Could you check a few things on this drawing? It's one solid part, dimensions in mm from its lowest x, y, z. A direction names the side the tool comes from. Round coordinates to 2 decimals unless told otherwise and drop trailing zeros. Write each loop counter-clockwise with the first axis right and the second up, starting at its lowest first coordinate (ties: lowest second). Pieces come first, ordered by that corner, then holes. Notation, with made-up numbers: (35.5, -7.5) -> (74.5, -7.5) arc R24 cw to (74.5, 6.5) -> close; hole circle Ø1 at (39.5, 48.25). An arc over 180 degrees is marked (long way). Answer in a Markdown table with one row per item. Add a question column.
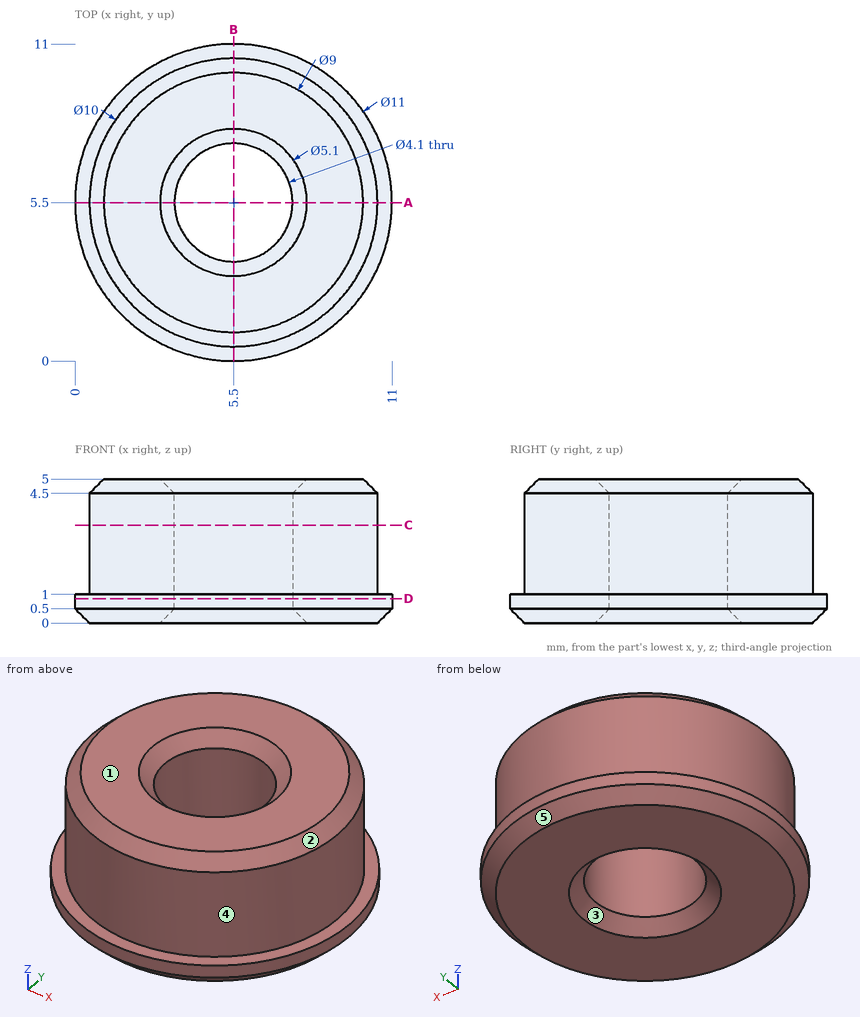
(1) I need wall thicknesses on L1, parallel to Y at x = 5.5, z = 1.6; L2, parallel to Y at x = 6.5, z = 4.4. Which ranges of each line are inside material? Lowest first, please.
(2) Suppose I cut it at A-A, the plane y = 5.5. Please give me the cut outline in (x, z), then the cut area to 3 significant figures.
(3) For P1, Ø1.5, axis at y = 7.5, z = 3.5, coming from the +X side; P2, Ø1.5, axis at y = 2.5, z = 3.5, coming from the +X side; P3, Ø2, axis at x = 4, z = 3, coming from the +Y side, each with a flat end and sliding along its axis, tell me the tip position at first contact or that it passes through.
(4) Suppose I cut it at C-C, the plane z = 3.4. Please give me the cut outline in (x, y).
(5) On a 3-axis mill with a long thin cutter (end or side, diameter ignored), from which of +Z, -Z, +X, -X, +Y, -Y can I reach the whole of each face in a straight line? I mean the marked faces 4 and 5. Say none if no direction works.
(6) If we mould it in two halves opening along Y, with no side actions, what happens to the marked faces 1, 2 and 3? For each: pulls with the +Y half, pulls with the -Y half, needs draft (parallel to the pull), parting line crosses it, or undercut.
(7) Suppose I cut it at D-D, the plane z = 0.85. Please give me the cut outline in (x, y), then the cut area to 3 significant figures.
Response:
| question | item | result |
|---|---|---|
| 1 | L1 | 0.5 to 3.45, 7.55 to 10.5 |
| 1 | L2 | 0.6 to 3.71, 7.29 to 10.4 |
| 2 | outline | (0, 0.5) -> (0.5, 0) -> (2.95, 0) -> (3.45, 0.5) -> (3.45, 4.5) -> (2.95, 5) -> (1, 5) -> (0.5, 4.5) -> (0.5, 1) -> (0, 1) -> close; (7.55, 0.5) -> (8.05, 0) -> (10.5, 0) -> (11, 0.5) -> (11, 1) -> (10.5, 1) -> (10.5, 4.5) -> (10, 5) -> (8.05, 5) -> (7.55, 4.5) -> close |
| 2 | area | 29.5 mm² |
| 3 | P1 | x = 10.34 |
| 3 | P2 | x = 9.97 |
| 3 | P3 | y = 10.47 |
| 4 | outline | circle Ø10 at (5.5, 5.5); hole circle Ø4.1 at (5.5, 5.5) |
| 5 | face 4 | +Z |
| 5 | face 5 | -Z |
| 6 | face 1 | needs draft |
| 6 | face 2 | parting line crosses it |
| 6 | face 3 | undercut |
| 7 | outline | circle Ø11 at (5.5, 5.5); hole circle Ø4.1 at (5.5, 5.5) |
| 7 | area | 81.8 mm² |
